```python
from build123d import *

# Parameters (mm, degrees)
F2_DEPTH = 25


# Not quite as in the source:
# - ends of sketch curves that miss each other by under 0.0002 mm in the source are joined


with BuildPart() as f2:
    # F1 (on face) → F2 (new body)
    with BuildSketch(Plane.XY):
        with BuildLine():
            ThreePointArc((-30.855476, 1.1181271498), (-28.0698825324, 0.6652748768), (-25.3272532308, 0))
            ThreePointArc((-25.3272532308, 0), (-9.3691647914, 9.3691647914), (0, 25.3272532308))
            ThreePointArc((0, 25.3272532308), (9.3691647914, 9.3691647914), (25.3272532308, 0))
            ThreePointArc((25.3272532308, 0), (9.3691647914, -9.3691647914), (0, -25.3272532308))
            ThreePointArc((0, -25.3272532308), (1.394661, -35.355339), (0, -45.3834247692))
            ThreePointArc((0, -45.3834247692), (58.7852402391, -63.6679197359), (51.8201256429, -2.5))
            Line((51.8201256429, -2.5), (30.855475, -2.5))
            Line((30.855475, -2.5), (30.855475, 2.5))
            Line((30.855475, 2.5), (51.8201256429, 2.5))
            ThreePointArc((51.8201256429, 2.5), (58.7852402391, 63.6679197359), (0, 45.3834247692))
            ThreePointArc((0, 45.3834247692), (-58.7852402391, 63.6679197359), (-51.8201256429, 2.5))
            Line((-51.8201256429, 2.5), (-30.855476, 2.5))
            Line((-30.855476, 2.5), (-30.855476, 1.1181271498))
        make_face()
        with BuildLine():
            ThreePointArc((-35.355339, 3.605339), (-57.8059793027, 57.8059793027), (-3.605339, 35.355339))
            Line((-3.605339, 35.355339), (-32.426206, 41.713026))
            ThreePointArc((-32.426206, 41.713026), (-40.3050867894, 40.3050861472), (-41.7130253526, 32.4262052983))
            Line((-41.7130253526, 32.4262052983), (-35.355339, 3.605339))
        make_face(mode=Mode.SUBTRACT)
    extrude(amount=F2_DEPTH)


solid = f2.part
```
The listing builds one solid part. Answer for the finished solid, in the listing's coordinates (mm). A direction names the side the tool comes from. Give positions to 0.01 mm unless a question says otherwise; leave off trailing zeros. Write each loop counter-clockwise with the first axis right and the second up, starting at its lowest first coordinate (ties: lowest second). Pieces come first, ordered by that corner, then holes. Notation, with made-up numbers: M 63,10.25 L 71,10.25 A11 cw 71,27.25 Z; hole C 64,43.5 d6. An arc over 180 degrees is marked long. Write each question's results on one line, items separated by ' | '.
Q1. Section B-B, the plane y = 16 is taken. Write down the section's boundary in (x, z), then the cut area to 3 significant figures.
Output values:
outline: M -66.6,0 L -60.52,0 L -60.52,25 L -66.6,25 Z; M -38.09,0 L -4.12,0 L -4.12,25 L -38.09,25 Z; M 4.12,0 L 66.6,0 L 66.6,25 L 4.12,25 Z | area: 2,560 mm2
Q2. Section D-D, the plane z = 9.75 is taken. Write down the section's boundary in (x, y), then the cut area to 3 significant figures.
Output values:
outline: M -51.82,2.5 L -30.86,2.5 L -30.86,1.12 A36.75 cw -25.33,0 A36.75 ccw 0,25.33 A36.75 ccw 25.33,0 A36.75 ccw 0,-25.33 A36.75 cw 0,-45.38 A36.75 ccw long 51.82,-2.5 L 30.86,-2.5 L 30.86,2.5 L 51.82,2.5 A36.75 ccw long 0,45.38 A36.75 ccw long Z; hole M -41.71,32.43 A7 cw -32.43,41.71 L -3.61,35.36 A31.75 ccw long -35.36,3.61 Z | area: 10,300 mm2
Q3. Section C-C, the plane x = -5.5 is taken. Write down the section's boundary in (y, z).
Output values:
outline: M 13.93,0 L 35.77,0 L 35.77,25 L 13.93,25 Z; M 46.16,0 L 56.78,0 L 56.78,25 L 46.16,25 Z
Q4. For a pull along Y with two mould halves and no side action, classify faces 1 (the cylindrical face through (1.394, -35.213, 12.325)), 2 (the flat face through (15, 17, 25)), 3 (the cylindrical face through (-28.109, 0.673, 12.325)) as released by +Y, released by -Y, zero draft, split by the parting line, or undercut.
Output values:
face 1: undercut | face 2: zero draft | face 3: released by -Y
Q5. Section A-A, the plane x = -38 is taken. Write down the section's boundary in (y, z) (3 decimals), then the cut area to 3 significant figures.
Output values:
outline: M 2.5,0 L 3.716,0 L 3.716,25 L 2.5,25 Z; M 15.594,0 L 41.837,0 L 41.837,25 L 15.594,25 Z; M 66.995,0 L 72.01,0 L 72.01,25 L 66.995,25 Z | area: 812 mm2
Q6. Flat-ended cylindrical pins translate along their axes: P1, Ø2, axis at x = -25, z = 15.5, coming from the +Y side; P2, Ø3, axis at y = -50, z = 5.5, coming from the -X side; P3, Ø1.5, axis at y = 19, z = 14.5, coming from the -X side. Find the tip coordinate at first contact, or state that the pin passes through.
Output values:
P1: y = 70.89 | P2: x = 1.04 | P3: x = -68.63
Q7. A tool of negligible diameter and unlimited length cuts with its end or side. For faces 4 (the flat face through (41, 2.5, 12)), 5 (the flat face through (-41, 2.5, 12)), 6 (the flat face through (15, 17, 0)), 7 (the flat face through (-17.81, 38.49, 12.32)), from which of +Z, -Z, +X, -X, +Y, -Y can it reach the whole face along a straight path? Write none if from no direction.
Output values:
face 4: +Z, -Z, +X | face 5: +Z, -Z, -X, -Y | face 6: -Z, +X, -X, +Y, -Y | face 7: +Z, -Z
Q8. Consider L1, parallel to X at y = 12, z = 18.5; L2, parallel to X at y = 49.5, z = 20; L3, parallel to Y at x = 37, z = 5.25. Determine where each line is inside the solid, lowest interval first. Write a range as from..to.
Output values:
L1: -63.73..-56.86, -37.21..-6.98, 6.98..63.73 | L2: -69.27..-63.78, -6.93..-1.44, 1.44..69.27 | L3: -72.07..-2.5, 2.5..72.07
